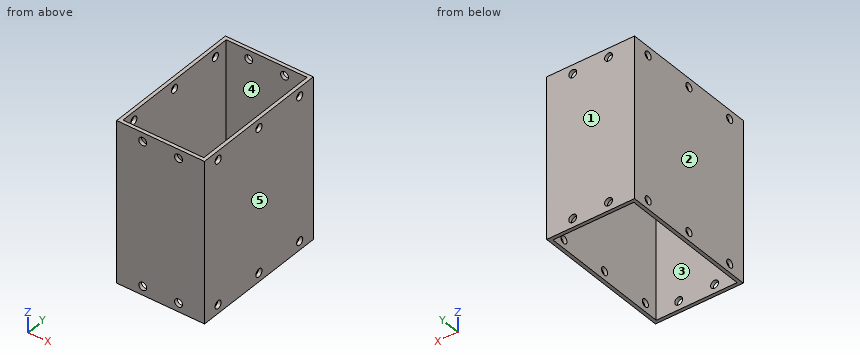
```python
from build123d import *

# Parameters (mm, degrees)
SKETCH1_W                      = 50
SKETCH1_H                      = 80
SKETCH1_W_2                    = 46
SKETCH1_H_2                    = 76
BOSS_EXTRUDE1_DEPTH            = 91.6
M4_CLEARANCE_HOLE1_D           = 4.5
M4_CLEARANCE_HOLE1_ON_FACE_2_D = 4.5
M4_CLEARANCE_HOLE1_ON_FACE_3_D = 4.5
M4_CLEARANCE_HOLE1_ON_FACE_4_D = 4.5


with BuildPart() as part:
    # Sketch1 → Boss-Extrude1 (new body)
    with BuildSketch(Plane.XY.offset(60)):
        Rectangle(SKETCH1_W, SKETCH1_H)
        Rectangle(SKETCH1_W_2, SKETCH1_H_2, mode=Mode.SUBTRACT)
    extrude(amount=BOSS_EXTRUDE1_DEPTH)

    # M4 Clearance Hole1 (through all)
    with Locations(Plane(origin=(25, 30, 65), x_dir=(0, 1, 0), z_dir=(1, 0, 0))):
        with Locations((0, 0), (-30, 0), (-60, 0), (-60, 81.6), (-30, 81.6), (0, 81.6)):
            Hole(M4_CLEARANCE_HOLE1_D / 2)

    # M4 Clearance Hole1 on face 2 (through all)
    with Locations(Plane(origin=(10.2, -40, 65), x_dir=(0, 0, -1), z_dir=(0, -1, 0))):
        with Locations((0, 0), (0, -20.4), (-81.6, -20.4), (-81.6, 0)):
            Hole(M4_CLEARANCE_HOLE1_ON_FACE_2_D / 2)

    # M4 Clearance Hole1 on face 3 (through all)
    with Locations(Plane(origin=(-25, -30, 65), x_dir=(0, 0, -1), z_dir=(-1, 0, 0))):
        with Locations((0, 0), (0, -60), (0, -30), (-81.6, -60), (-81.6, -30), (-81.6, 0)):
            Hole(M4_CLEARANCE_HOLE1_ON_FACE_3_D / 2)

    # M4 Clearance Hole1 on face 4 (through all)
    with Locations(Plane(origin=(10.2, 40, 65), x_dir=(0, 0, 1), z_dir=(0, 1, 0))):
        with Locations((0, 0), (0, -20.4), (81.6, 0), (81.6, -20.4)):
            Hole(M4_CLEARANCE_HOLE1_ON_FACE_4_D / 2)


solid = part.part
```
Verification items for the finished model (mm, model axes). Face numbers are marked on the shaded views. A direction names the side the tool comes from. Coordinates: 2 decimals unless noted, no trailing zeros. Order: outer loops, then holes, each group sorted by start corner. A loop starts at its lowest first (then second) coordinate and runs counter-clockwise, first axis right, second up. Notation, with made-up numbers: (73, 63.5) - (83, 63.5) arc R33 cw to (83, 101.5) - close; hole circle Ø8 at (62.5, 79). An arc over 180 degrees is marked (long way). Return JSON: item names as keys, results as strings.
(1) Section check A-A, the plane y = -6.5. Record the cut outline in (x, z).
Filled sheet:
{"outline": "(-25, 60) - (-23, 60) - (-23, 151.6) - (-25, 151.6) - close; (23, 60) - (25, 60) - (25, 151.6) - (23, 151.6) - close"}
(2) Mould release check, pull along X, two halves, no side actions. Record for the marked faces 1, 2 and 3: pulls with the +X half, pulls with the -X half, needs draft (parallel to the pull), parting line crosses it, or undercut.
Filled sheet:
{"face 1": "needs draft", "face 2": "pulls with the -X half", "face 3": "undercut"}
(3) Section check B-B, the plane x = -17. Record the cut outline in (y, z), and give its area (3 significant figures).
Filled sheet:
{"outline": "(-40, 60) - (-38, 60) - (-38, 151.6) - (-40, 151.6) - close; (38, 60) - (40, 60) - (40, 151.6) - (38, 151.6) - close", "area": "366 mm^2"}
(4) Section check D-D, the plane y = -30. Record the cut outline in (x, z), and give its area (3 significant figures).
Filled sheet:
{"outline": "(-25, 60) - (-23, 60) - (-23, 62.75) - (-25, 62.75) - close; (-25, 67.25) - (-23, 67.25) - (-23, 144.35) - (-25, 144.35) - close; (-25, 148.85) - (-23, 148.85) - (-23, 151.6) - (-25, 151.6) - close; (23, 60) - (25, 60) - (25, 62.75) - (23, 62.75) - close; (23, 67.25) - (25, 67.25) - (25, 144.35) - (23, 144.35) - close; (23, 148.85) - (25, 148.85) - (25, 151.6) - (23, 151.6) - close", "area": "330 mm^2"}
(5) Section check C-C, the plane z = 141. Record the cut outline in (x, y), and give its area (3 significant figures).
Filled sheet:
{"outline": "(-25, -40) - (25, -40) - (25, 40) - (-25, 40) - close; hole (-23, -38) - (23, -38) - (23, 38) - (-23, 38) - close", "area": "504 mm^2"}
(6) Thickness scan on line 1 along Z through (x, y) = (23.4, 0); line 2 along X through (y, z) = (20.5, 88); line 3 along Y through (x, z) = (15, 136). Record the ranges inside material, lowest first.
Filled sheet:
{"line 1": "z = 60 to 62.75, 67.25 to 144.35, 148.85 to 151.6", "line 2": "x = -25 to -23, 23 to 25", "line 3": "y = -40 to -38, 38 to 40"}
(7) Access from +Z, -Z, +X, -X, +Y, -Y to the whole of each face (thin tool, end or side, straight path). Record for the marked faces 4 and 5.
Filled sheet:
{"face 4": "+Z, -Z", "face 5": "+Z, -Z, +X, +Y, -Y"}
